Geometry: final body of the model. Coordinates: model frame, mm. A direction names the side the tool comes from. Round coordinates to 2 decimals unless told otherwise and drop trailing zeros. Write each loop counter-clockwise with the first axis right and the second up, starting at its lowest first coordinate (ties: lowest second). Pieces come first, ordered by that corner, then holes. Notation, with made-up numbers: (16.5, -10.5) - (36.5, -10.5) arc R11 ccw to (36.5, 0.5) - close; hole circle Ø9 at (6.25, -19). An arc over 180 degrees is marked (long way). Write each question's results on one line, items separated by ' | '.
from build123d import *

# Parameters (mm, degrees)
ESBO_O1_R                  = 10
RESSALTO_EXTRUS_O1_DEPTH   = 40
CORTE_EXTRUS_O1_DEPTH      = 79.102496759
CORTE_EXTRUS_O1_DEPTH_BACK = 79.102496759
ESBO_O2_W                  = 20
ESBO_O2_H                  = 35


with BuildPart() as part:
    # Esboço1 → Ressalto-extrusão1 (new body)
    with BuildSketch(Plane.XY):
        with BuildLine():
            Line((15, -30), (15, -24))
            Line((15, -24), (-15, -24))
            Line((-15, -24), (-15, -30))
            Line((-15, -30), (-40, -30))
            Line((-40, -30), (-40, -15))
            Line((-40, -15), (-20, -15))
            Line((-20, -15), (-20, 0))
            ThreePointArc((-20, 0), (0, 20), (20, 0))
            Line((20, 0), (20, -15))
            Line((20, -15), (40, -15))
            Line((40, -15), (40, -30))
            Line((40, -30), (15, -30))
        make_face()
        Circle(ESBO_O1_R, mode=Mode.SUBTRACT)
    extrude(amount=-RESSALTO_EXTRUS_O1_DEPTH)

    # Esboço2 → Corte-extrusão1 (cut, two sides: drawn at the far end of the back side and taken through both)
    with BuildSketch(Plane.ZY.offset(20).offset(-CORTE_EXTRUS_O1_DEPTH_BACK)):
        with Locations((-20, 2.5)):
            Rectangle(ESBO_O2_W, ESBO_O2_H)
    extrude(amount=CORTE_EXTRUS_O1_DEPTH + CORTE_EXTRUS_O1_DEPTH_BACK, mode=Mode.SUBTRACT)


solid = part.part
Q1. Access query for faces 4 (the flat face through (-4, 10, -30)), 5 (the flat face through (-15, -27, -20)), 6 (the flat face through (-20, -8, -35)). Directions: +Z, -Z, +X, -X, +Y, -Y. A direction counts if a zero-diameter tool reaches every point of the face in a straight line with its end or side. Return the directions, or none.
Answer block:
face 4: +X, -X, +Y | face 5: +Z, -Z, -Y | face 6: +Z, -Z, -X, +Y
Q2. Section query B-B, the plane y = -14. Return loops of the section in (x, z).
Answer block:
outline: (-20, -40) - (20, -40) - (20, -30) - (-20, -30) - close; (-20, -10) - (20, -10) - (20, 0) - (-20, 0) - close
Q3. Section query D-D, the plane y = 1.5. Return loops of the section in (x, z), plus the area to 3 significant figures.
Answer block:
outline: (-19.94, -40) - (-9.89, -40) - (-9.89, -30) - (-19.94, -30) - close; (-19.94, -10) - (-9.89, -10) - (-9.89, 0) - (-19.94, 0) - close; (9.89, -40) - (19.94, -40) - (19.94, -30) - (9.89, -30) - close; (9.89, -10) - (19.94, -10) - (19.94, 0) - (9.89, 0) - close | area: 402 mm2
Q4. Section query C-C, the plane x = 0. Return loops of the section in (y, z), plus the area to 3 significant figures.
Answer block:
outline: (-24, -40) - (-10, -40) - (-10, -30) - (-15, -30) - (-15, -10) - (-10, -10) - (-10, 0) - (-24, 0) - close; (10, -40) - (20, -40) - (20, -30) - (10, -30) - close; (10, -10) - (20, -10) - (20, 0) - (10, 0) - close | area: 660 mm2
Q5. Ray query, line 1 along Y through (x, z) = (0, -8); line 2 along Z through (x, y) = (18, 4.5); line 3 along X through (y, z) = (-25, -2). Return the intervals inside material, ascending.
Answer block:
line 1: -24 to -10, 10 to 20 | line 2: -40 to -30, -10 to 0 | line 3: -40 to -15, 15 to 40
Q6. Pin query (flat end, axial travel): pin 1 (8 mm diameter, centred on x = -5, z = -6, fed in from +Y) (3 decimals); pin 2 (12 mm diameter, centred on x = 13, z = -20.5, fed in from +Y); pin 3 (5 mm diameter, centred on y = -6, z = -33.5, fed in from +X); pin 4 (5 mm diameter, centred on x = -17, y = 13, fed in from +Z). Return the tip coordinate at first contact, or that it passes through.
Answer block:
pin 1: y = 19.975 | pin 2: y = -15 | pin 3: x = 20 | pin 4: z = 0
Q7. Section query A-A, the plane z = -7. Return loops of the section in (x, y), plus the area to 3 significant figures.
Answer block:
outline: (-40, -30) - (-15, -30) - (-15, -24) - (15, -24) - (15, -30) - (40, -30) - (40, -15) - (20, -15) - (20, 0) arc R20 ccw to (-20, 0) - (-20, -15) - (-40, -15) - close; hole circle Ø20 at (0, 0) | area: 1,930 mm2
Q8. Mould query, pull axis X, two halves, no side actions, for faces 1 (the flat face through (20, -7, -35)), 2 (the cylindrical face through (-2.17, -9.76, -34.93)), 3 (the flat face through (-40, -23, -20)). Classes: pulls with the +X half, pulls with the -X half, needs draft (parallel to the pull), parting line crosses it, or undercut.
Answer block:
face 1: pulls with the +X half | face 2: undercut | face 3: pulls with the -X half
